```python
from build123d import *

# Parameters (mm, degrees)
F0_R     = 9
F1_DEPTH = 5


with BuildPart() as f1:
    # F0 (on Top) → F1 (new body)
    with BuildSketch(Plane.XY):
        with BuildLine():
            Line((20, 80), (0, 80))
            Line((0, 80), (-20, 80))
            ThreePointArc((-20, 80), (-34.142136, 74.142136), (-40, 60))
            Line((-40, 60), (-40, -60))
            ThreePointArc((-40, -60), (-34.142136, -74.142136), (-20, -80))
            Line((-20, -80), (20, -80))
            ThreePointArc((20, -80), (34.142136, -74.142136), (40, -60))
            Line((40, -60), (40, 60))
            ThreePointArc((40, 60), (34.142136, 74.142136), (20, 80))
        make_face()
        with Locations((0, -65)):
            Circle(F0_R, mode=Mode.SUBTRACT)
        with BuildLine():
            ThreePointArc((25.25, -23.25), (24.664214, -24.664214), (23.25, -25.25))
            Line((23.25, -25.25), (-23.25, -25.25))
            ThreePointArc((-23.25, -25.25), (-24.664214, -24.664214), (-25.25, -23.25))
            Line((-25.25, -23.25), (-25.25, 23.25))
            ThreePointArc((-25.25, 23.25), (-24.664214, 24.664214), (-23.25, 25.25))
            Line((-23.25, 25.25), (23.25, 25.25))
            ThreePointArc((23.25, 25.25), (24.664214, 24.664214), (25.25, 23.25))
            Line((25.25, 23.25), (25.25, -23.25))
        make_face(mode=Mode.SUBTRACT)
        with BuildLine():
            ThreePointArc((9, 65), (-6.363961, 58.636039), (0, 74))
            ThreePointArc((0, 74), (6.363961, 71.363961), (9, 65))
        make_face(mode=Mode.SUBTRACT)
    extrude(amount=F1_DEPTH)


solid = f1.part
```
Input: part model. Units: mm. Frame: model coordinates. A direction names the side the tool comes from. Coordinates: 2 decimals unless noted, no trailing zeros. Write each loop counter-clockwise with the first axis right and the second up, starting at its lowest first coordinate (ties: lowest second). Pieces come first, ordered by that corner, then holes. Notation, with made-up numbers: (-31.5, -32.75) -> (-10.5, -32.75) arc R36 cw to (-10.5, 6.25) -> close; hole circle Ø4 at (13, 61.5). An arc over 180 degrees is marked (long way). Write each question's results on one line, items separated by ' | '.
Item 1: Section query A-A on y = 18. Return loops of the section in (x, z), plus the area to 4 significant figures.
Conclusion:
outline: (-40, 0) -> (-25.25, 0) -> (-25.25, 5) -> (-40, 5) -> close; (25.25, 0) -> (40, 0) -> (40, 5) -> (25.25, 5) -> close | area: 147.5 mm^2
Item 2: Pin query (flat end, axial travel): pin 1 Ø3 at (x, z) = (24, 2.5) entering from +Y; pin 2 Ø3 at (x, y) = (7.5, -26) entering from -Z. Return the tip coordinate at first contact, or that it passes through.
Conclusion:
pin 1: stops at y = 79.84 | pin 2: stops at z = 0
Item 3: Section query B-B on z = 2.5. Return loops of the section in (x, y), plus the area to 3 significant figures.
Conclusion:
outline: (-40, -60) arc R20 ccw to (-20, -80) -> (20, -80) arc R20 ccw to (40, -60) -> (40, 60) arc R20 ccw to (20, 80) -> (-20, 80) arc R20 ccw to (-40, 60) -> close; hole (-25.25, -23.25) arc R2 ccw to (-23.25, -25.25) -> (23.25, -25.25) arc R2 ccw to (25.25, -23.25) -> (25.25, 23.25) arc R2 ccw to (23.25, 25.25) -> (-23.25, 25.25) arc R2 ccw to (-25.25, 23.25) -> close; hole circle Ø18 at (0, -65); hole circle Ø18 at (0, 65) | area: 9,400 mm^2
Item 4: Material intervals for probe 1 along Y at (x, z) = (0, 3.7); probe 2 along X at (y, z) = (-0.5, 1.4); probe 3 along Y at (x, z) = (21, 3.6), sorted ascending.
Conclusion:
probe 1: y = -80 to -74, -56 to -25.25, 25.25 to 56, 74 to 80 | probe 2: x = -40 to -25.25, 25.25 to 40 | probe 3: y = -79.97 to -25.25, 25.25 to 79.97
Item 5: Section query C-C on x = -32. Return loops of the section in (y, z), plus the area to 3 significant figures.
Conclusion:
outline: (-76, 0) -> (76, 0) -> (76, 5) -> (-76, 5) -> close | area: 760 mm^2
Item 6: Set-up query: faces 1 (the flat face through (0, -25.25, 2)), 2 (the flat face through (26, 1, 5)). Return all of +Z, -Z, +X, -X, +Y, -Y with unobstructed straight access to the full face (end or side cutting, diameter ignored); none if empty.
Conclusion:
face 1: +Z, -Z | face 2: +Z, +X, -X, +Y, -Y
Item 7: Mould query, pull axis Y, two halves, no side actions, for faces 3 (the cylindrical face through (-1.951, -73.786, 2.465)), 4 (the cylindrical face through (-33.986, 74.297, 2.465)), 5 (the cylindrical face through (-34.297, -73.986, 2.465)), 6 (the flat face through (0, 25.25, 2)). Classes: +Y half, -Y half, draft (parallel to the pull), parting line (faces both ways), or undercut.
Conclusion:
face 3: undercut | face 4: +Y half | face 5: -Y half | face 6: undercut
Item 8: Section query D-D on y = -65. Return loops of the section in (x, z), plus the area to 3 significant figures.
Conclusion:
outline: (-39.36, 0) -> (-9, 0) -> (-9, 5) -> (-39.36, 5) -> close; (9, 0) -> (39.36, 0) -> (39.36, 5) -> (9, 5) -> close | area: 304 mm^2
